from build123d import *

# Parameters (mm, degrees)
SKETCH1_R           = 1.5
BOSS_EXTRUDE1_DEPTH = 3.175


with BuildPart() as part:
    # Sketch1 → Boss-Extrude1 (new body)
    with BuildSketch(Plane(origin=(0, 0, 0), x_dir=(1, 0, 0), z_dir=(0, 1, 0))):
        with BuildLine():
            Line((-5.08, 0), (-5.08, -5.9309))
            Line((-5.08, -5.9309), (-3.175, -5.9309))
            Line((-3.175, -5.9309), (-3.175, -11.9761))
            Line((-3.175, -11.9761), (3.175, -11.9761))
            Line((3.175, -11.9761), (3.175, -5.9309))
            Line((3.175, -5.9309), (5.08, -5.9309))
            Line((5.08, -5.9309), (5.08, 0))
            ThreePointArc((5.08, 0), (0, 5.08), (-5.08, 0))
        make_face()
        with Locations(Location((0, 0, 0), (0, 0, 270))):
            Circle(SKETCH1_R, mode=Mode.SUBTRACT)
    extrude(amount=BOSS_EXTRUDE1_DEPTH)


solid = part.part
Read the model definition and answer for the solid it produces. Units are mm, in the model's axes. A direction names the side the tool comes from. Coordinates: 2 decimals unless noted, no trailing zeros. Order: outer loops, then holes, each group sorted by start corner. A loop starts at its lowest first (then second) coordinate and runs counter-clockwise, first axis right, second up. Notation, with made-up numbers: (-15.75, 67) -> (24.25, 67) arc R18 ccw to (24.25, 102) -> close; hole circle Ø9 at (28.25, 37.25). An arc over 180 degrees is marked (long way). Answer as a JSON object with one key per item and string values.
1) A cutting plane is placed at D-D, the plane x = 1.25. Determine the outline of the cut face in (y, z) (3 decimals), plus the area to 3 significant figures.
Model answer:
{"outline": "(0, -4.924) -> (3.175, -4.924) -> (3.175, -0.829) -> (0, -0.829) -> close; (0, 0.829) -> (3.175, 0.829) -> (3.175, 11.976) -> (0, 11.976) -> close", "area": "48.4 mm²"}
2) Each of these flat-tipped pins is pushed along its axis until it touches: pin 1 (1.5 mm diameter, centred on x = 1, y = 1, fed in from -Z); pin 2 (1.6 mm diameter, centred on y = 2, z = 9, fed in from +X) (3 decimals); pin 3 (1.5 mm diameter, centred on x = 4, y = 2, fed in from +Z); pin 4 (4 mm diameter, centred on x = 0, z = 0, fed in from +Y) (3 decimals). Where does it stop, or does it pass through?
Model answer:
{"pin 1": "stops at z = -5.07", "pin 2": "stops at x = 3.175", "pin 3": "stops at z = 5.93", "pin 4": "stops at y = 3.175"}
3) A cutting plane is placed at B-B, the plane y = 1.5. Determine the outline of the cut face in (x, z) (3 decimals).
Model answer:
{"outline": "(-5.08, 0) arc R5.08 ccw to (5.08, 0) -> (5.08, 5.931) -> (3.175, 5.931) -> (3.175, 11.976) -> (-3.175, 11.976) -> (-3.175, 5.931) -> (-5.08, 5.931) -> close; hole circle Ø3 at (0, 0)"}
4) A cutting plane is placed at A-A, the plane x = 0. Determine the outline of the cut face in (y, z) (3 decimals), plus the area to 3 significant figures.
Model answer:
{"outline": "(0, -5.08) -> (3.175, -5.08) -> (3.175, -1.5) -> (0, -1.5) -> close; (0, 1.5) -> (3.175, 1.5) -> (3.175, 11.976) -> (0, 11.976) -> close", "area": "44.6 mm²"}
5) Consider line 1 along X through (y, z) = (1.7, 8) (3 decimals); line 2 along Z through (x, y) = (-0.25, 2.9); line 3 along X through (y, z) = (0.2, 0.25). Determine where each line is inside the solid, lowest interval first. Write a range as from..to.
Model answer:
{"line 1": "x = -3.175..3.175", "line 2": "z = -5.07..-1.48, 1.48..11.98", "line 3": "x = -5.08..-1.48, 1.48..5.08"}
6) A tool of negligible diameter and unlimited length cuts with its end or side. For faces 1 (the face through (5.08, 2, 3)), 2 (the face through (4, 2, 5.931)), 3 (the face through (-3.175, 2, 9)), from which of +Z, -Z, +X, -X, +Y, -Y can it reach the whole face along a straight path? Write none if from no direction.
Model answer:
{"face 1": "+Z, -Z, +X, +Y, -Y", "face 2": "+Z, +X, +Y, -Y", "face 3": "+Z, -X, +Y, -Y"}
7) A cutting plane is placed at C-C, the plane z = 9.5. Determine the outline of the cut face in (x, y) (3 decimals), plus the area to 3 significant figures.
Model answer:
{"outline": "(-3.175, 0) -> (3.175, 0) -> (3.175, 3.175) -> (-3.175, 3.175) -> close", "area": "20.2 mm²"}
8) The mould has two halves that part along Z. Classify faces 4 (the face through (0, 3.175, 3)), 5 (the face through (0.45, 1.57, 1.43)), 6 (the face through (-4, 2, 5.931)): released by +Z, released by -Z, zero draft, split by the parting line, or undercut.
Model answer:
{"face 4": "zero draft", "face 5": "undercut", "face 6": "released by +Z"}
